```python
from build123d import *

# Parameters (mm, degrees)
SKETCH4_OUTSIDE_W   = 62.634
SKETCH4_OUTSIDE_H   = 62.634
SKETCH4_OUTSIDE_W_2 = 33.924910587
SKETCH4_OUTSIDE_H_2 = 10
CUT_EXTRUDE1_DEPTH  = 60
SKETCH9_R           = 6
BOSS_EXTRUDE1_DEPTH = 14


with BuildPart() as part:
    # Sketch1 → Revolve1 (revolve)
    with BuildSketch(Plane(origin=(0, 0, 0), x_dir=(1, 0, 0), z_dir=(0, 1, 0)), mode=Mode.PRIVATE) as revolve1_sk:
        Polygon((57.735849057, -1.8), (57.735849057, 6.2), (-117.46468802, 6.2), (-117.46468802, 10.2), (-122.264150943, 10.2), (-122.264150943, -1.8), align=None)
    revolve(revolve1_sk.sketch.rotate(Axis((-122.264150943, 0, 1.8), (1, 0, 0)), 180), axis=Axis((-122.264150943, 0, 1.8), (1, 0, 0)))

    # Sketch4 outside → Cut-Extrude1 (cut)
    with BuildSketch(Plane(origin=(57.735849057, 0, 0), x_dir=(0, 0, -1), z_dir=(1, 0, 0))):
        with Locations((-1.8, 0)):
            Rectangle(SKETCH4_OUTSIDE_W, SKETCH4_OUTSIDE_H)
        with Locations((-4.763294948, 0)):
            Rectangle(SKETCH4_OUTSIDE_W_2, SKETCH4_OUTSIDE_H_2, mode=Mode.SUBTRACT)
    extrude(amount=-CUT_EXTRUDE1_DEPTH, mode=Mode.SUBTRACT)

    # Sketch9 → Boss-Extrude1 (add)
    with BuildSketch(Plane(origin=(0, 5, 0), x_dir=(1, 0, 0), z_dir=(0, 1, 0))):
        with Locations(Location((38.985849057, -1.8, 0), (0, 0, 270))):
            Circle(SKETCH9_R)
    extrude(amount=BOSS_EXTRUDE1_DEPTH)


solid = part.part
```
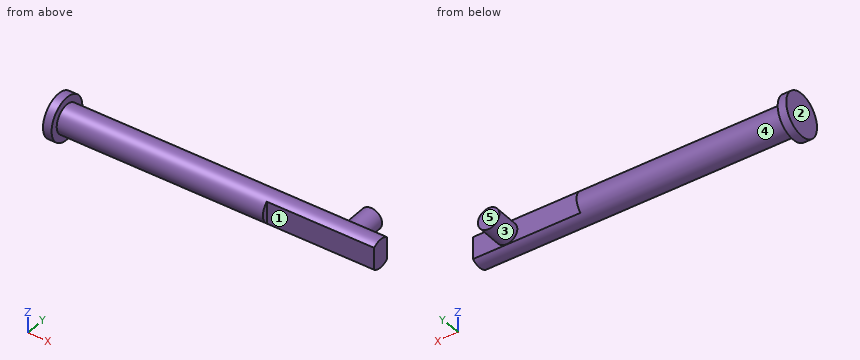
The model under review builds one solid part; all positions refer to its coordinate system, in mm. Face numbers are marked on the shaded views. A direction names the side the tool comes from. Round coordinates to 2 decimals unless told otherwise and drop trailing zeros. Write each loop counter-clockwise with the first axis right and the second up, starting at its lowest first coordinate (ties: lowest second). Pieces come first, ordered by that corner, then holes. Notation, with made-up numbers: (9, -30) - (43, -30) arc R28 ccw to (43, -3) - close; hole circle Ø5 at (66.25, 68.25). An arc over 180 degrees is marked (long way). Answer as CSV lines item,"result". Start each with the question number.
(1) We need section D-D on y = 15. State the section outline as (x, z) points, plus the area to 3 significant figures.
(2) We need section A-A on y = 0. State the section outline as (x, z) points, plus the area to 3 significant figures.
(3) We need section B-B on z = 1.8. State the section outline as (x, y) points.
(4) Draft analysis for pull direction X (two halves, no side actions). For the marked faces 1, 2 and 3, state which applies: pulls with the +X half, pulls with the -X half, needs draft (parallel to the pull), parting line crosses it, or undercut.
(5) We need section C-C on x = -80.5. State the section outline as (y, z) points.
(6) For the marked faces 4 and 5, list the 3-axis set-ups (+Z, -Z, +X, -X, +Y, -Y) from which the entire face can be reached by the end or side of a thin tool; tool diameter is ignored.
(7) For pin 1 Ø10 at (x, z) = (41, 1.5) entering from -Y; pin 2 Ø1.5 at (y, z) = (-6, 2) entering from +X; pin 3 Ø2 at (x, z) = (-26, 2) entering from -Y, all flat-tipped, find the tip position at first contact; note any pin that passes through.
(8) To check wall thickness, follow line 1 (X direction, y = 6, z = -8.25); line 2 (X direction, y = 10, z = -0.25); line 3 (Y direction, x = -8.5, z = 8.25). State the ranges of each line that lie inside material, in increasing order.
Worked answers:
1,outline,"circle Ø12 at (38.99, 1.8)"
1,area,"113 mm²"
2,outline,"(-122.26, -10.2) - (-117.46, -10.2) - (-117.46, -6.2) - (57.74, -6.2) - (57.74, 9.8) - (-117.46, 9.8) - (-117.46, 13.8) - (-122.26, 13.8) - close"
2,area,"2,920 mm²"
3,outline,"(-122.26, -12) - (-117.46, -12) - (-117.46, -8) - (-2.26, -8) - (-2.26, -5) - (57.74, -5) - (57.74, 5) - (44.99, 5) - (44.99, 19) - (32.99, 19) - (32.99, 5) - (-2.26, 5) - (-2.26, 8) - (-117.46, 8) - (-117.46, 12) - (-122.26, 12) - close"
4,face 1,"needs draft"
4,face 2,"pulls with the -X half"
4,face 3,"undercut"
5,outline,"circle Ø16 at (0, 1.8)"
6,face 4,"none"
6,face 5,"+Z, -Z, +X, -X, +Y"
7,pin 1,"y = -5"
7,pin 2,"x = -2.26"
7,pin 3,"y = -8"
8,line 1,"-122.26 to -117.46"
8,line 2,"-122.26 to -117.46, 33.35 to 44.62"
8,line 3,"-4.73 to 4.73"
